The listing builds one solid part. Answer for the finished solid, in the listing's coordinates (mm). A direction names the side the tool comes from. Round coordinates to 2 decimals unless told otherwise and drop trailing zeros. Write each loop counter-clockwise with the first axis right and the second up, starting at its lowest first coordinate (ties: lowest second). Pieces come first, ordered by that corner, then holes.
(1) A cutting plane is placed at D-D, the plane x = -30.5. Give the vertices of the cut face in (y, z), and give its area (3 significant figures).
(2) Find the intervals of material crossed by probe 1 along Z at (x, y) = (-20.5, 22); probe 2 along X at (y, z) = (-13, 30.5); probe 3 along Z at (x, y) = (0.5, 0.5), in increasing order.
(3) A cutting plane is placed at A-A, the plane y = 0. Give the vertices of the cut face in (x, z).
(4) Each of these flat-tipped pins is pushed along its axis until it touches: pin 1 Ø10 at (x, y) = (-37, 9.5) entering from +Z; pin 2 Ø3 at (y, z) = (16, 28.5) entering from +X. Where does it stop, or does it pass through?
(5) A cutting plane is placed at B-B, the plane x = 0. Give the vertices of the cut face in (y, z), and give its area (3 significant figures).
(6) A cutting plane is placed at C-C, the plane z = 31.5. Give the vertices of the cut face in (x, y).
(7) For faces 1 (the face through (-1, -33.597, 13)), 2 (the face through (-19.45, 0.86, 33.45)), determine the directions among +Z, -Z, +X, -X, +Y, -Y from which every point of the face is accessible in a straight line to the end or side of a thin tool.
from build123d import *

# Parameters (mm, degrees)
F0_W     = 101.13819
F0_H     = 67.194544
F1_DEPTH = 25.4
F2_R     = 19.468615
F3_DEPTH = 25.4
F5_DEPTH = 82.804


with BuildPart() as f1:
    # F0 (on Top) → F1 (new body)
    with BuildSketch(Plane.XY):
        Rectangle(F0_W, F0_H)
    extrude(amount=F1_DEPTH)

    # F2 (on face) → F3 (join)
    with BuildSketch(Plane.XY.offset(25.4)):
        Circle(F2_R)
    extrude(amount=F3_DEPTH)

    # F4 (on face) → F5 (cut)
    with BuildSketch(Plane.XZ.offset(33.597272)):
        Polygon((-19.627273, 46.297271), (20.550909, 34.578636), (20.550909, 51.608179), (-19.627273, 51.608179), align=None)
    extrude(amount=-F5_DEPTH, mode=Mode.SUBTRACT)


solid = f1.part
Solutions:
1. outline: (-33.6, 0) - (33.6, 0) - (33.6, 25.4) - (-33.6, 25.4) - close
1. area: 1,710 mm2
2. probe 1: z = 0 to 25.4
2. probe 2: x = -14.49 to 14.49
2. probe 3: z = 0 to 40.43
3. outline: (-50.57, 0) - (50.57, 0) - (50.57, 25.4) - (19.47, 25.4) - (19.47, 34.89) - (-19.47, 46.25) - (-19.47, 25.4) - (-50.57, 25.4) - close
4. pin 1: stops at z = 25.4
4. pin 2: stops at x = 12.99
5. outline: (-33.6, 0) - (33.6, 0) - (33.6, 25.4) - (19.47, 25.4) - (19.47, 40.57) - (-19.47, 40.57) - (-19.47, 25.4) - (-33.6, 25.4) - close
5. area: 2,300 mm2
6. outline: circle Ø38.94 at (0, 0)
7. face 1: +Z, -Z, +X, -X, -Y
7. face 2: +Z
